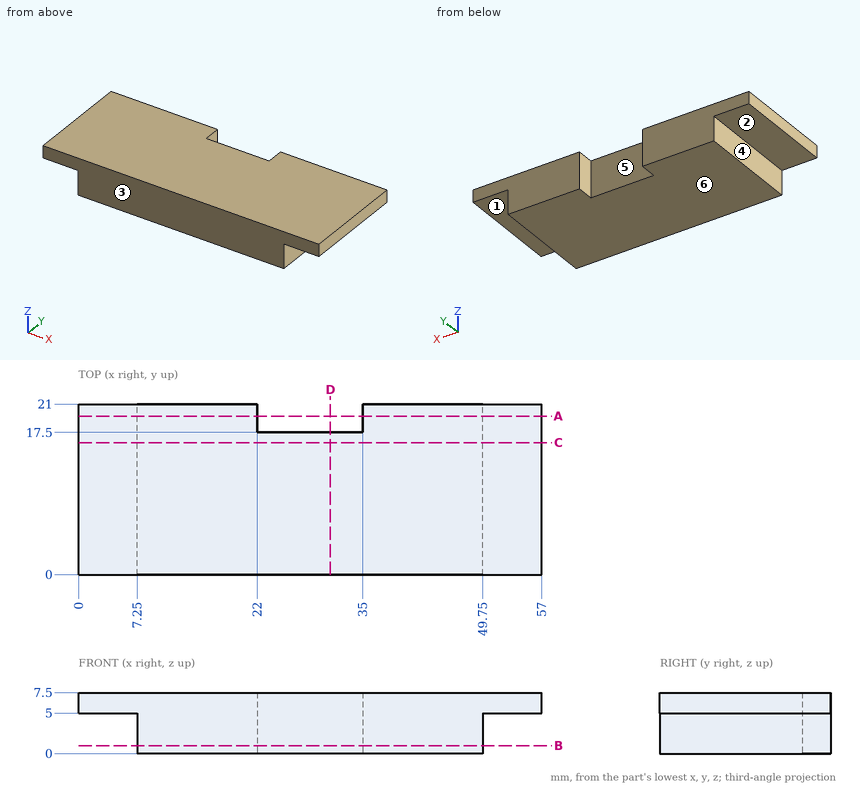
Answer from the drawing. Dimensions are ordinates in mm from the lowest x, y and z of the part. A direction names the side the tool comes from. Give positions to 0.01 mm unless a question says otherwise; leave off trailing zeros. Order: outer loops, then holes, each group sorted by start corner. A loop starts at its lowest first (then second) coordinate and runs counter-clockwise, first axis right, second up.
(1) Find section B-B (z = 1). Give the vertices of the cut face in (x, y), plus the area to 3 significant figures.
(2) For a pull along X with two mould halves and no side action, classify the marked faces 4, 5 and 6 as released by +X, released by -X, zero draft, split by the parting line, or undercut.
(3) For the marked faces 1, 2 and 3, determine the directions among +Z, -Z, +X, -X, +Y, -Y from which every point of the face is accessible in a straight line to the end or side of a thin tool.
(4) Straight lines are drawn through the part: L1, parallel to X at y = 19, z = 4.5; L2, parallel to Z at x = 54, y = 14; L3, parallel to X at y = 6.25, z = 1.75. For each, find the intervals that lie inside material, in ascending order.
(5) Find section A-A (y = 19.5). Give the vertices of the cut face in (x, z), plus the area to 4 significant figures.
(6) Find section D-D (x = 31). Give the vertices of the cut face in (y, z), plus the area to 3 significant figures.
(7) Given pin 1 (1.5 mm diameter, centred on y = 6.5, z = 3, fed in from +X); pin 2 (6 mm diameter, centred on x = 53, y = 12.5, fed in from -Z); pin 3 (2.5 mm diameter, centred on y = 13.5, z = 3.5, fed in from -X), each flat-ended and moving along its own axis, determine where each tip first touches the part or whether it passes through.
(8) Find section C-C (y = 16.25). Give the vertices of the cut face in (x, z), plus the area to 3 significant figures.
Result sheet:
1. outline: (7.25, 0) - (49.75, 0) - (49.75, 21) - (35, 21) - (35, 17.5) - (22, 17.5) - (22, 21) - (7.25, 21) - close
1. area: 847 mm2
2. face 4: released by -X
2. face 5: undercut
2. face 6: zero draft
3. face 1: -Z, +X, +Y, -Y
3. face 2: -Z, -X, +Y, -Y
3. face 3: +Z, -Z, +X, -X, -Y
4. L1: x = 7.25 to 22, 35 to 49.75
4. L2: z = 5 to 7.5
4. L3: x = 7.25 to 49.75
5. outline: (0, 5) - (7.25, 5) - (7.25, 0) - (22, 0) - (22, 7.5) - (0, 7.5) - close; (35, 0) - (49.75, 0) - (49.75, 5) - (57, 5) - (57, 7.5) - (35, 7.5) - close
5. area: 257.5 mm2
6. outline: (0, 0) - (17.5, 0) - (17.5, 7.5) - (0, 7.5) - close
6. area: 131 mm2
7. pin 1: stops at x = 49.75
7. pin 2: stops at z = 5
7. pin 3: stops at x = 7.25
8. outline: (0, 5) - (7.25, 5) - (7.25, 0) - (49.75, 0) - (49.75, 5) - (57, 5) - (57, 7.5) - (0, 7.5) - close
8. area: 355 mm2
